Here's how the part is built. I have some questions about the finished solid (model axes, mm). Give positions to 0.01 mm unless a question says otherwise; leave off trailing zeros. Write each loop counter-clockwise with the first axis right and the second up, starting at its lowest first coordinate (ties: lowest second). Pieces come first, ordered by that corner, then holes. Notation, with made-up numbers: (21, 21) - (51, 21) arc R26 ccw to (51, 43) - close; hole circle Ø4 at (4.5, 6). An arc over 180 degrees is marked (long way). Write each question's results on one line, items separated by ' | '. Start each with the question number.
Item 1: Please list where these lines run through material, in increasing order: line 1 along Z through (x, y) = (0.55, 10); line 2 along Y through (x, z) = (1.5, 10); line 3 along Z through (x, y) = (0.55, 9).
Item 2: Suppose I cut it at B-B on y = 25. List the corners of the cut face in (x, z) for me.
Item 3: Suppose I cut it at D-D on y = 10. List the corners of the cut face in (x, z) for me, then the cut area to 3 significant figures.
Item 4: Suppose I cut it at A-A on z = 5. List the corners of the cut face in (x, y) for me, then the cut area to 3 significant figures.
Item 5: Will these pins go through, and if not, where does the flat tip stop? P1, Ø0.6, axis at x = 0.5, z = 27.5, coming from the +Y side; P2, Ø2.5, axis at y = 10, z = 25, coming from the -X side (3 decimals).
Item 6: Suppose I cut it at C-C on x = 1.4. List the corners of the cut face in (y, z) for me, then the cut area to 3 significant figures.
Autodesk Inventor part; units mm, degrees
ref_plane "YZ Plane" through (0, 0, 0) normal (1, 0, 0) x (0, 1, 0)
ref_plane "XZ Plane" through (0, 0, 0) normal (0, 1, 0) x (-1, 0, 0)
ref_plane "XY Plane" through (0, 0, 0) normal (0, 0, 1) x (1, 0, 0)
sketch "スケッチ1" plane through (0, 0, 0) normal (1, 0, 0) x (0, 1, 0)
  line L0 (0, 0) -> (50, 0)
  line L1 (50, 0) -> (50, 20)
  line L2 (50, 20) -> (0, 20)
  line L3 (0, 20) -> (0, 0)
  line L4 (0, 0) -> (20, 0)
  line L5 (20, 0) -> (20, 30)
  line L6 (20, 30) -> (0, 30)
  line L7 (0, 30) -> (0, 0)
  point P0 (0, 20)
  point P1 (20, 20)
  point P2 (20, 0)
  point P3 (20, 0)
  dimension "d0" = 20
  dimension "d1" = 20
  dimension "d2" = 30
  dimension "d3" = 30
extrude "押し出し1" add sketch "スケッチ1" along normal blind 2
sketch "スケッチ2" plane through (2, 0, 0) normal (1, 0, 0) x (0, 0, -1)
  line L0 (-30, 20) -> (-30, 0)
  line L1 (-30, 10) -> (0, 10) construction
  line L2 (0, 0) -> (0, 50)
  line L3 (0, 50) -> (-20, 50)
  line L4 (-10, 50) -> (-10, 0) construction
  line L5 (-30, 0) -> (0, 0)
  point P0 (-25, 10)
  point P1 (-5, 10)
  point P2 (-10, 25)
  point P3 (-10, 45)
  dimension "d6" = 20
  dimension "d7" = 5
  dimension "d8" = 20
  dimension "d9" = 5
hole "穴1" at (2, 10, 25) at (2, 10, 5) at (2, 25, 10) at (2, 45, 10) direction (-1, 0, 0) diameter 3.2 end through all
properties part number "FrameJointL2020" material "アルミニウム 6061"
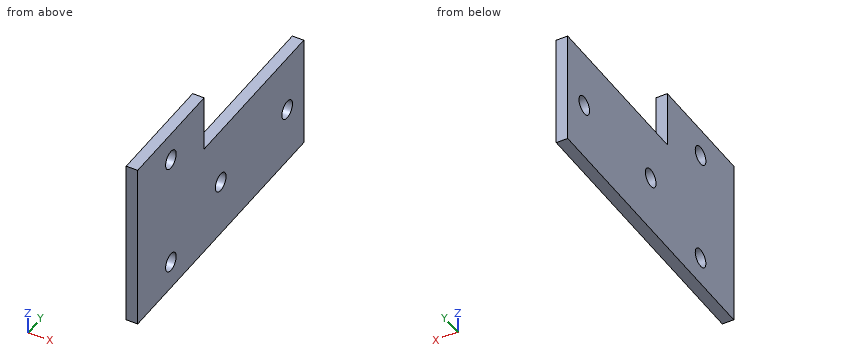
Checked values:
1) line 1: z = 0 to 3.4, 6.6 to 23.4, 26.6 to 30 | line 2: y = 0 to 23.4, 26.6 to 43.4, 46.6 to 50 | line 3: z = 0 to 3.75, 6.25 to 23.75, 26.25 to 30
2) outline: (0, 0) - (2, 0) - (2, 8.4) - (0, 8.4) - close; (0, 11.6) - (2, 11.6) - (2, 20) - (0, 20) - close
3) outline: (0, 0) - (2, 0) - (2, 3.4) - (0, 3.4) - close; (0, 6.6) - (2, 6.6) - (2, 23.4) - (0, 23.4) - close; (0, 26.6) - (2, 26.6) - (2, 30) - (0, 30) - close | area: 47.2 mm^2
4) outline: (0, 0) - (2, 0) - (2, 8.4) - (0, 8.4) - close; (0, 11.6) - (2, 11.6) - (2, 50) - (0, 50) - close | area: 93.6 mm^2
5) P1: stops at y = 20 | P2: passes through
6) outline: (0, 0) - (50, 0) - (50, 20) - (20, 20) - (20, 30) - (0, 30) - close; hole circle Ø3.2 at (10, 5); hole circle Ø3.2 at (10, 25); hole circle Ø3.2 at (25, 10); hole circle Ø3.2 at (45, 10) | area: 1,170 mm^2
